The model under review builds one solid part; all positions refer to its coordinate system, in mm. Coordinates: 2 decimals unless noted, no trailing zeros. Order: outer loops, then holes, each group sorted by start corner. A loop starts at its lowest first (then second) coordinate and runs counter-clockwise, first axis right, second up. Notation, with made-up numbers: (51, 13.25) -> (101, 13.25) arc R12 ccw to (101, 28.25) -> close; hole circle Ø3 at (-19, -5). An arc over 180 degrees is marked (long way). Use one line per item in the form item = value.
from build123d import *

# Parameters (mm, degrees)
F0_R          = 4.191
F0_R_2        = 2.921
F1_DEPTH      = 111.125
F3_DEPTH      = 0.79375
F3_DEPTH_BACK = 0.79375
F4_COUNT      = 3
F5_D          = 6.35
F5_DEPTH      = 111.1260001


# Not quite as in the source:
# - a length typed as a fraction of an inch, garbled in the dataset ("3 / 203.2 mm" for 3/8 in), is restored


with BuildPart() as f1:
    # F0 (on Top) → F1 (new body)
    with BuildSketch(Plane.XY):
        Circle(F0_R)
        Circle(F0_R_2, mode=Mode.SUBTRACT)
    extrude(amount=F1_DEPTH)

    # F2 (on Front) → F3 (join, two sides)
    with BuildSketch(Plane.XZ) as f3_sk:
        with BuildLine():
            ThreePointArc((52.1055692807, 22.1924969852), (16.1288428569, 60.3431066176), (3.05240741, 111.125))
            Line((3.05240741, 111.125), (3.05240741, -12.6199012697))
            Line((3.05240741, -12.6199012697), (52.1055692807, -12.6199012697))
            Line((52.1055692807, -12.6199012697), (52.1055692807, 22.1924969852))
        make_face()
        Polygon((52.1055692807, -12.6199012697), (3.05240741, -12.6199012697), (52.1055692807, -53.9700498879), align=None)
    extrude(amount=F3_DEPTH)
    extrude(f3_sk.sketch, amount=-F3_DEPTH_BACK)

    # F4: F1 ×3 about axis
    f4_axis = Axis((0, 0, 24.9059423804), (0, 0, -1))


with BuildPart() as f1_1:
    add(f1.part)
    for i in range(1, F4_COUNT):
        add(f1.part.rotate(f4_axis, i * 360 / F4_COUNT))

    # F5 (through all, one way)
    with BuildSketch(Plane(origin=(0, 0, 0), x_dir=(1, 0, 0), z_dir=(0, 0, -1))):
        with Locations((0, 0)):
            Circle(F5_D / 2)
    extrude(amount=-F5_DEPTH, mode=Mode.SUBTRACT)


solid = f1_1.part
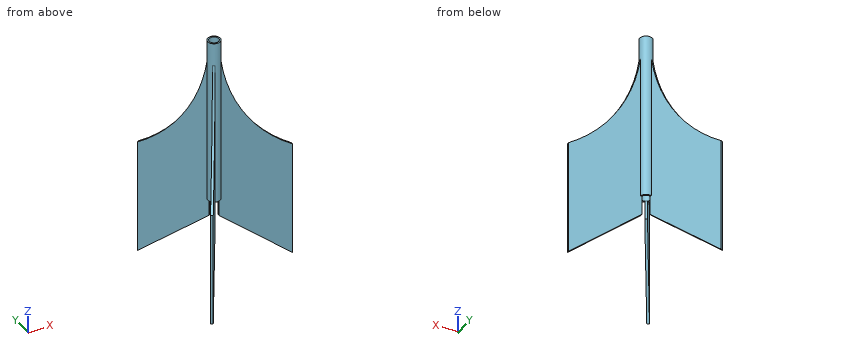
Item 1: We need section A-A (z = 25). Write out the cut boundary in (x, y) (3 decimals).
Results found:
outline = (-24.629, -41.071) -> (-23.254, -41.865) -> (-1.37, -3.961) arc R4.191 ccw to (4.115, -0.794) -> (47.883, -0.794) -> (47.883, 0.794) -> (4.115, 0.794) arc R4.191 ccw to (-1.37, 3.961) -> (-23.254, 41.865) -> (-24.629, 41.071) -> (-2.745, 3.167) arc R4.191 ccw to (-2.745, -3.167) -> close; hole circle Ø6.35 at (0, 0)
Item 2: To check wall thickness, follow L1, parallel to Y at x = 0, z = 38 (3 decimals); L2, parallel to Y at x = 17, z = 35.5; L3, parallel to Y at x = -7.5, z = 21. State the ranges of each line that lie inside material, in increasing order. Write a range as from..to.
Results found:
L1 = -4.191..-3.175, 3.175..4.191
L2 = -0.79..0.79
L3 = -14.58..-11.4, 11.4..14.58
Item 3: We need section D-D (x = 47). Write out the cut boundary in (y, z).
Results found:
outline = (-0.79, -49.67) -> (0.79, -49.67) -> (0.79, 25.63) -> (-0.79, 25.63) -> close
Item 4: We need section C-C (x = 13.5). Write out the cut boundary in (y, z), plus the area to 3 significant figures.
Results found:
outline = (-0.79, -21.43) -> (0.79, -21.43) -> (0.79, 65.43) -> (-0.79, 65.43) -> close
area = 138 mm²
Item 5: Clearance check with flat-ended pins moving along their axes: pin 1 (1.5 mm diameter, centred on y = 15, z = -21.5, fed in from -X); pin 2 (4 mm diameter, centred on y = 26.5, z = -27, fed in from -X); pin 3 (3.5 mm diameter, centred on x = 0.5, y = -3, fed in from -Z). State where each tip first meets the part, or that it passes through.
Results found:
pin_1 = -10.01
pin_2 = -17.37
pin_3 = -13.15
Item 6: We need section B-B (z = 98.5). Write out the cut boundary in (x, y) (3 decimals).
Results found:
outline = circle Ø8.382 at (0, 0); hole circle Ø6.35 at (0, 0)
